Build history of the part. All positions in model axes, mm. Face numbers are marked on the shaded views. A direction names the side the tool comes from. Round coordinates to 2 decimals unless told otherwise and drop trailing zeros. Write each loop counter-clockwise with the first axis right and the second up, starting at its lowest first coordinate (ties: lowest second). Pieces come first, ordered by that corner, then holes.
Item 1: Wall check: probe 1 along X at (y, z) = (29, -19); probe 2 along X at (y, z) = (70.5, 19); probe 3 along Z at (x, y) = (-0.5, 31). Give the ranges that are in metal, low to high.
Item 2: Band-saw the part on D-D, the plane x = 1.5. Write the cut outline in (y, z) (3 decimals).
Item 3: Band-saw the part on C-C, the plane x = 12. Write the cut outline in (y, z) (3 decimals).
Item 4: 3-axis set-ups, long thin cutter, end or side, ignore diameter. For the marked faces 1 and 2: which of +Z, -Z, +X, -X, +Y, -Y reach the whole face in a straight line?
Item 5: Band-saw the part on B-B, the plane z = 32.5. Write the cut outline in (x, y).
Item 6: Mould opens along X. For the marked faces 3, 4 and 5 say: +X half, -X half, draft (parallel to the pull), parting line (faces both ways), or undercut.
Item 7: Drop flat-ended pins along their axis: pin 1 Ø8 at (x, z) = (10, -35.5) entering from +Y; pin 2 Ø9.5 at (y, z) = (83, 24) entering from -X; pin 3 Ø10 at (y, z) = (60.5, -9.5) entering from -X (1 decimal); pin 4 Ø1 at (x, z) = (-5, 8) entering from +Y. Give the stop position or say it passes through.
Item 8: Band-saw the part on A-A, the plane y = 20. Write the cut outline in (x, z), then the cut area to 3 significant figures.
Autodesk Inventor part; units mm, degrees
ref_plane "YZ Plane" through (0, 0, 0) normal (1, 0, 0) x (0, 1, 0)
ref_plane "XZ Plane" through (0, 0, 0) normal (0, 1, 0) x (-1, 0, 0)
ref_plane "XY Plane" through (0, 0, 0) normal (0, 0, 1) x (1, 0, 0)
sketch "Sketch1" plane through (0, 0, 0) normal (0, 1, 0) x (-1, 0, 0)
  line L0 (0, 42.5) -> (0, -42.5)
  line L1 (15, 0) -> (-15, 0)
  line L2 (0, 42.5) -> (15, 42.5)
  line L3 (15, 42.5) -> (15, -42.5)
  line L4 (15, -42.5) -> (-15, -42.5)
  line L5 (0, 42.5) -> (-15, 42.5)
  line L6 (-15, 42.5) -> (-15, -42.5)
  point P0 (0, 0)
  point P1 (0, 0)
  point P2 (0, 0)
extrude "Extrusion1" add sketch "Sketch1" along normal blind 95
fillet "Fillet1" radius 25 1 edges at (-7.5, 0, 42.5)
sketch "Sketch2" plane through (15, 0, -42.5) normal (1, 0, 0) x (0, 0, -1)
  arc A0 (-85, 25) -> (-60, 0) centre (-60, 25) ccw
  line L0 (-60, 0) -> (0, 0)
  line L1 (0, 0) -> (0, 95)
  line L2 (-85, 95) -> (0, 95)
  line L3 (-85, 25) -> (-85, 95)
  circle A1 centre (-60, 25) radius 10
  line L4 (0, 0) -> (0, 12.5)
  line L5 (0, 0) -> (0, 95)
  line L6 (0, 12.5) -> (-25, 12.5)
  line L7 (0, 12.5) -> (0, 27.5)
  line L8 (0, 27.5) -> (0, 40)
  line L9 (0, 40) -> (-40, 40)
  line L10 (0, 27.5) -> (-25, 27.5)
  arc A2 (-25, 27.5) -> (-25, 12.5) centre (-25, 20) ccw
  point P0 (-42.5, 0)
  dimension "d5" = 20
  dimension "d6" = 12.5
  dimension "d7" = 25
  dimension "d8" = 15
  dimension "d9" = 12.5
  dimension "d10" = 40
extrude "Extrusion2" cut sketch "Sketch2" against normal up to next contours L6 A2 L10 L1 | A1
sketch "Sketch3" plane through (15, 95, 42.5) normal (1, 0, 0) x (0, 0, -1)
  line L0 (85, -82.5) -> (60, -82.5)
  arc A0 (60, -67.5) -> (60, -82.5) centre (60, -75) ccw
  line L1 (60, -67.5) -> (85, -67.5)
  line L2 (85, -67.5) -> (85, 0)
  line L3 (0, 0) -> (85, 0)
  line L4 (0, -70) -> (0, 0)
  arc A1 (0, -70) -> (25, -95) centre (25, -70) ccw
  line L5 (25, -95) -> (85, -95)
  line L6 (85, -95) -> (85, -82.5)
  circle A2 centre (25, -70) radius 10
  line L7 (25, -70) -> (25, 29)
  line L8 (25, -70) -> (-1.9532, 30.5909)
  line L9 (25, -70) -> (10.765, -16.8741)
  circle A3 centre (10.765, -16.8741) radius 6.5
  circle A4 centre (10.765, -16.8741) radius 20
  line L10 (0, 0) -> (85, 0)
  line L11 (85, 0) -> (0, 0)
  point P0 (42.5, -95)
  dimension "d13" = 15
  dimension "d14" = 55
  dimension "d15" = 13
  dimension "d17" = 40
extrude "Extrusion3" cut sketch "Sketch3" against normal up to next contours A3 L8 | L8 A3
extrude "Extrusion4" cut sketch "Sketch3" against normal blind 6 contours A4 L4 | L4 A4 L3 L8 A3 | L8 A3 L3 A4 L7 | L3 L8 A4 | A4 L7 | A4 L8 L3
fillet "Fillet2" radius 15 1 edges at (0, 95, 42.5)
sketch "Sketch5" plane through (15, 0, -42.5) normal (0, 0, -1) x (-1, 0, 0)
  line L0 (30, 12.5) -> (0, 12.5)
  line L1 (0, 0) -> (0, 12.5)
  line L2 (0, 0) -> (30, 0)
  line L3 (30, 0) -> (30, 12.5)
  line L4 (0, 0) -> (7.5, 0)
  line L5 (7.5, 0) -> (7.5, 40)
  line L6 (7.5, 40) -> (22.5, 40)
  line L7 (22.5, 40) -> (22.5, 0)
  point P0 (15, 0)
  dimension "d28" = 7.5
  dimension "d29" = 40
  dimension "d30" = 15
extrude "Extrusion6" cut sketch "Sketch5" against normal blind 40 contours L7 L2 L5 L0 | L0 L5 L6 L7
sketch "Sketch6" plane through (15, 0, 17.5) normal (1, 0, 0) x (0, 0, -1)
  arc A0 (-25, 61.2702) -> (-3.4989, 95) centre (-14.235, 78.1259) ccw
  line L0 (-25, 25) -> (-25, 61.2702)
  arc A1 (-25, 25) -> (0, 0) centre (0, 25) ccw
  line L1 (0, 0) -> (60, 0)
  line L2 (60, 0) -> (60, 12.5)
  line L3 (60, 12.5) -> (35, 12.5)
  arc A2 (35, 27.5) -> (35, 12.5) centre (35, 20) ccw
  line L4 (35, 27.5) -> (60, 27.5)
  line L5 (60, 27.5) -> (60, 95)
  line L6 (-3.4989, 95) -> (60, 95)
  circle A3 centre (0, 25) radius 10
  line L7 (-14.235, 78.1259) -> (5.765, 78.1259)
  line L8 (60, 40) -> (60, 27.5)
  line L9 (60, 0) -> (60, 40)
  line L10 (60, 40) -> (20, 40)
  line L11 (60, 40) -> (20, 40)
  line L12 (20, 40) -> (20, 54)
  circle A4 centre (62, 110) radius 70
  point P0 (17.5, 0)
  point P1 (4.2372, 70.4594)
  point P2 (60, 40.0286)
  dimension "d33" = 140
extrude "Extrusion7" cut sketch "Sketch6" against normal up to next contours A0 L6 L5 A4
sketch "Sketch7" plane through (-15, 0, -42.5) normal (-1, 0, 0) x (0, 0, 1)
  circle A0 centre (60, 25) radius 10
  circle A1 centre (74.235, 78.1259) radius 6.5
  arc A2 (0, 40.0286) -> (55.7628, 70.4594) centre (-2, 110) ccw
  line L0 (0, 27.5) -> (0, 40.0286)
  line L1 (0, 27.5) -> (25, 27.5)
  arc A3 (25, 12.5) -> (25, 27.5) centre (25, 20) ccw
  line L2 (25, 12.5) -> (0, 12.5)
  line L3 (0, 0) -> (0, 12.5)
  line L4 (0, 0) -> (60, 0)
  arc A4 (60, 0) -> (85, 25) centre (60, 25) ccw
  line L5 (85, 25) -> (85, 80)
  arc A5 (85, 80) -> (70, 95) centre (70, 80) ccw
  line L6 (63.4989, 95) -> (70, 95)
  circle A6 centre (74.235, 78.1259) radius 20
  arc A7 (63.4989, 95) -> (55.7628, 70.4594) centre (74.235, 78.1259) ccw
  point P0 (42.5, 0)
  dimension "d36" = 40
extrude "Extrusion8" cut sketch "Sketch7" against normal blind 6 contours A1 | A6 L6 A5 L5 | A6 L5 A5 L6
fillet "Fillet3" radius 15 1 edges at (0, 95, 20.9989)
sketch "Sketch8" plane through (-7.5, 40, -42.5) normal (0, -1, 0) x (1, 0, 0)
  line L0 (0, 0) -> (0, 40)
  line L1 (0, 40) -> (15, 40)
  line L2 (15, 0) -> (15, 40)
  line L3 (15, 40) -> (15, 0)
  line L4 (15, 0) -> (0, 0)
  line L5 (0, 0) -> (0, 40)
  point P0 (7.5, 42.5)
extrude "Extrusion9" cut sketch "Sketch8" against normal up to next
sketch "Sketch9" plane through (9, 95, 42.5) normal (1, 0, 0) x (0, 0, -1)
  circle A0 centre (25, -70) radius 10
  arc A1 (29.2372, -24.5406) -> (85, -54.9714) centre (87, 15) ccw
  arc A2 (0, -33.7298) -> (29.2372, -24.5406) centre (10.765, -16.8741) ccw
  line L0 (0, -70) -> (0, -33.7298)
  arc A3 (0, -70) -> (25, -95) centre (25, -70) ccw
  line L1 (25, -95) -> (85, -95)
  line L2 (85, -95) -> (85, -82.5)
  line L3 (85, -82.5) -> (60, -82.5)
  arc A4 (60, -67.5) -> (60, -82.5) centre (60, -75) ccw
  line L4 (60, -67.5) -> (85, -67.5)
  line L5 (85, -67.5) -> (85, -54.9714)
  line L6 (10.765, -16.8741) -> (29.2372, -16.8741)
  circle A5 centre (29.2372, -16.8741) radius 10
  point P0 (42.5, -95)
  dimension "d42" = 20
extrude "Extrusion10" cut sketch "Sketch9" along normal blind 10 contours A2 A5 A1 | A1 A5 A2
sketch "Sketch10" plane through (-9, 0, -42.5) normal (-1, 0, 0) x (0, 0, 1)
  circle A0 centre (74.235, 78.1259) radius 6.5
  arc A1 (69.5996, 95) -> (55.6931, 85.6222) centre (69.5996, 80) ccw
  arc A2 (55.6931, 85.6222) -> (55.7628, 70.4594) centre (74.235, 78.1259) ccw
  arc A3 (55.7628, 70.4594) -> (85, 61.2702) centre (74.235, 78.1259) ccw
  line L0 (85, 80) -> (85, 61.2702)
  arc A4 (85, 80) -> (70, 95) centre (70, 80) ccw
  line L1 (69.5996, 95) -> (70, 95)
  line L2 (74.235, 78.1259) -> (42.5, 78.1259)
  circle A5 centre (54.235, 78.1259) radius 10
  point P0 (42.5, 0)
  dimension "d45" = 20
extrude "Extrusion11" cut sketch "Sketch10" along normal blind 10 contours A5 A3 A2 L2 | L2 A2 A1 A5 | L2 A5 A1 A2 | A2 A3 A5 L2
properties part number "FIGURA3_U3_MINIPROYECTO"
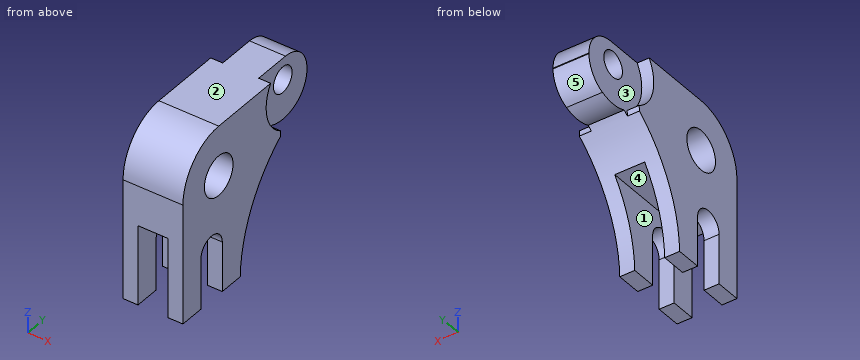
Results:
1. probe 1: x = -15 to -7.5, 7.5 to 15
1. probe 2: x = -9 to 9
1. probe 3: z = -2.5 to 9.5, 25.5 to 42.5
2. outline: (0, -2.5) - (54, -2.5) arc R70 cw to (70.459, 13.263) arc R20 ccw to (85.622, 13.193) arc R15 ccw to (95, 27.1) - (95, 27.5) arc R15 ccw to (80, 42.5) - (25, 42.5) arc R25 ccw to (0, 17.5) - close; hole circle Ø20 at (25, 17.5); hole circle Ø13 at (78.126, 31.735)
3. outline: (0, -42.5) - (12.5, -42.5) - (12.5, -17.5) arc R7.5 cw to (27.5, -17.5) - (27.5, -42.5) - (40.029, -42.5) arc R70 cw to (68.251, 11.687) arc R10 cw to (68.188, 14.379) arc R20 cw to (61.27, 42.5) - (25, 42.5) arc R25 ccw to (0, 17.5) - close; hole circle Ø20 at (25, 17.5)
4. face 1: -Z, +Y, -Y
4. face 2: +Z, +X, -X, +Y, -Y
5. outline: (-15, 5) - (15, 5) - (15, 58.14) - (9, 58.14) - (9, 71.67) - (-9, 71.67) - (-9, 58.14) - (-15, 58.14) - close; (-9, 84.58) - (9, 84.58) - (9, 94.14) - (-9, 94.14) - close
6. face 3: -X half
6. face 4: undercut
6. face 5: draft
7. pin 1: stops at y = 41.22
7. pin 2: stops at x = -9
7. pin 3: passes through
7. pin 4: stops at y = 64.27
8. outline: (-15, -10) - (-7.5, -10) - (-7.5, -2.5) - (7.5, -2.5) - (7.5, -10) - (15, -10) - (15, 8.84) - (-15, 8.84) - close; (-15, 26.16) - (15, 26.16) - (15, 41.99) - (-15, 41.99) - close
8. area: 928 mm2
